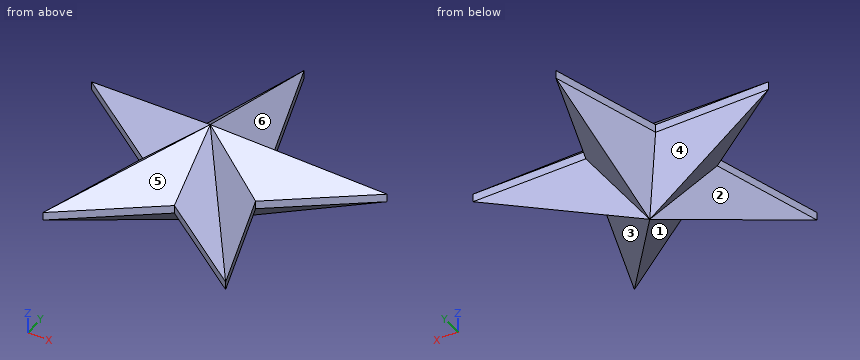
from build123d import *

# Parameters (mm, degrees)
F1_DEPTH = 25
F2_SIZE  = 23


with BuildPart() as f1:
    # F0 (on Top) → F1 (new body)
    with BuildSketch(Plane.XY):
        Polygon((16.8215913544, 23.1529342137), (0, 74.9244689941), (-16.8215913544, 23.1529342137), align=None)
        Polygon((-16.8215913544, 23.1529342137), (-71.2574044668, 23.1529342137), (-27.2179065562, -8.8436339303), align=None)
        Polygon((27.2179065562, -8.8436339303), (71.2574044668, 23.1529342137), (16.8215913544, 23.1529342137), align=None)
        Polygon((-27.2179065562, -8.8436339303), (-44.0394979106, -60.6151687108), (0, -28.6186005667), align=None)
        Polygon((0, -28.6186005667), (44.0394979106, -60.6151687108), (27.2179065562, -8.8436339303), align=None)
        Polygon((16.8215913544, 23.1529342137), (-16.8215913544, 23.1529342137), (-27.2179065562, -8.8436339303), (0, -28.6186005667), (27.2179065562, -8.8436339303), align=None)
    extrude(amount=F1_DEPTH)

    # F2
    f2_edges = [f1.edges().sort_by_distance(p)[0] for p in [
        (8.410796, 49.038702, 25),
        (-8.410796, 49.038702, 25),
        (-44.039498, 23.152934, 25),
        (-49.237656, 7.15465, 25),
        (-35.628702, -34.729401, 25),
        (-22.019749, -44.616885, 25),
        (22.019749, -44.616885, 25),
        (35.628702, -34.729401, 25),
        (49.237656, 7.15465, 25),
        (44.039498, 23.152934, 25),
    ]]
    chamfer(f2_edges, length=F2_SIZE)

    # F3: F1 across plane


with BuildPart() as f1_1:
    add(f1.part)
    add(f1.part.mirror(Plane.XY))


solid = f1_1.part
Model file for the job. Use its own axes, mm. Face numbers are marked on the shaded views. A direction names the side the tool comes from. Coordinates: 2 decimals unless noted, no trailing zeros. Order: outer loops, then holes, each group sorted by start corner. A loop starts at its lowest first (then second) coordinate and runs counter-clockwise, first axis right, second up. Notation, with made-up numbers: (72, 42) -> (103, 42) arc R17 cw to (103, 59) -> close; hole circle Ø10 at (-21, -2). An arc over 180 degrees is marked (long way). Return JSON: item names as keys, results as strings. Group by question number.
Item 1: Pull direction X, two halves, no side cores. Call the marked faces 4, 5 and 6: pulls with the +X half, pulls with the -X half, needs draft (parallel to the pull), parting line crosses it, or undercut.
Item 2: Saw through at A-A on x = 36. Write the cut outline in (y, z), then the cut area to 3 significant figures.
Item 3: Tool access for the marked faces 1, 2 and 3: list every direction of +Z, -Z, +X, -X, +Y, -Y with a clear straight run to the whole face (end or side of a thin tool).
Item 4: Saw through at B-B on z = 11. Write the cut outline in (x, y).
Item 5: Flat gauge pins, fed straight in: P1, Ø3, axis at x = 8, y = 43, coming from the -Z side; P2, Ø10, axis at x = -40.5, z = -2, coming from the +Y side; P3, Ø5, axis at y = 36, z = -10, coming from the +X side. Where does each tip first touch, or does it go through?
Item 6: Saw through at D-D on x = -6.5. Write the cut outline in (y, z), then the cut area to 3 significant figures.
Item 7: Saw through at C-C on y = 13.5. Write the cut outline in (x, z), then the cut area to 3 significant figures.
Item 8: Wall check: line 1 along Z through (x, y) = (14, 31.5); line 2 along Y through (x, z) = (22, -6); line 3 along Y through (x, z) = (-28.5, 11). Give the ranges that are in metal, low to high. Write a range as [from, to].
Values found:
{
 "1": {"face 4": "needs draft", "face 5": "undercut", "face 6": "pulls with the +X half"},
 "2": {"outline": "(-54.77, -2) -> (-49.55, -6.23) -> (-35.87, -2) -> (-35.87, 2) -> (-49.55, 6.23) -> (-54.77, 2) -> close; (-2.46, -2) -> (11.7, -13.46) -> (23.15, -2) -> (23.15, 2) -> (11.7, 13.46) -> (-2.46, 2) -> close", "area": "551 mm2"},
 "3": {"face 1": "-Z, -Y", "face 2": "-Z, -X", "face 3": "-Z, +X"},
 "4": {"outline": "(-43.56, 14.15) -> (-16.64, -5.41) -> (-26.92, -37.05) -> (0, -17.49) -> (26.92, -37.05) -> (16.64, -5.41) -> (43.56, 14.15) -> (10.28, 14.15) -> (0, 45.8) -> (-10.28, 14.15) -> close"},
 "5": {"P1": "stops at z = -5.76", "P2": "stops at y = 23.15", "P3": "stops at x = 6.99"},
 "6": {"outline": "(-33.34, -2) -> (-8.95, -21.74) -> (-2.11, -19.62) -> (2.11, -23.04) -> (8.95, -16.21) -> (54.92, -2) -> (54.92, 2) -> (8.95, 16.21) -> (2.11, 23.04) -> (-2.11, 19.62) -> (-8.95, 21.74) -> (-33.34, 2) -> close", "area": "2,150 mm2"},
 "7": {"outline": "(-57.97, -2) -> (-41.55, -11.65) -> (-9.81, -11.65) -> (0, -20.98) -> (9.81, -11.65) -> (41.55, -11.65) -> (57.97, -2) -> (57.97, 2) -> (41.55, 11.65) -> (9.81, 11.65) -> (0, 20.98) -> (-9.81, 11.65) -> (-41.55, 11.65) -> (-57.97, 2) -> close", "area": "2,570 mm2"},
 "8": {"line 1": "z = [-2.1, 2.1]", "line 2": "y = [-39.66, 19.15]", "line 3": "y = [3.21, 14.15]"}
}
